Can you work these out from the model? Positions are in its coordinate system, mm. Face numbers are marked on the shaded views. A direction names the side the tool comes from. Give positions to 0.01 mm unless a question says otherwise; leave off trailing zeros. Write each loop counter-clockwise with the first axis right and the second up, starting at its lowest first coordinate (ties: lowest second). Pieces come first, ordered by that corner, then holes. Notation, with made-up numbers: M 86,-10.5 L 133,-10.5 A19 cw 133,26.5 Z; hole C 84,8.25 d2. An arc over 180 degrees is marked long. Use CSV: the item, a comma, the result in double quotes. Start each with the question number.
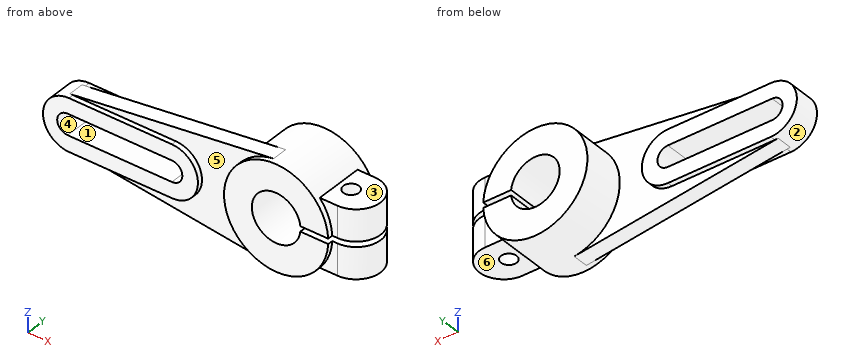
from build123d import *

# Parameters (mm, degrees)
BOSS_EXTRUDE1_DEPTH = 7.5
BOSS_EXTRUDE2_DEPTH = 4.5
BOSS_EXTRUDE3_START = 28.5
BOSS_EXTRUDE3_DEPTH = 36
BOSS_EXTRUDE4_START = 23.5
SKETCH1_5_W         = 16.939679335
SKETCH1_5_H         = 18
BOSS_EXTRUDE4_DEPTH = 28
FILLET1_RADIUS      = 14
FILLET1_LENGTH      = 18
FILLET2_RADIUS      = 14
FILLET2_LENGTH      = 18
SKETCH2_R           = 4.5
CUT_EXTRUDE1_DEPTH  = 146.8618303


with BuildPart() as part:
    # Sketch1 → Boss-Extrude1 (new, symmetric)
    with BuildSketch(Plane(origin=(0, 0, 0), x_dir=(1, 0, 0), z_dir=(0, 1, 0))):
        with BuildLine():
            Line((-119.21316455, -15), (-60, -15))
            ThreePointArc((-60, -15), (-45, 0), (-60, 15))
            Line((-60, 15), (-119.21316455, 15))
            ThreePointArc((-119.21316455, 15), (-134.21316455, 0), (-119.21316455, -15))
        make_face()
        with BuildLine():
            ThreePointArc((-120, 6), (-126, 0), (-120, -6))
            Line((-120, -6), (-60, -6))
            ThreePointArc((-60, -6), (-54, 0), (-60, 6))
            Line((-60, 6), (-120, 6))
        make_face(mode=Mode.SUBTRACT)
    extrude(amount=BOSS_EXTRUDE1_DEPTH, both=True)

    # Sketch1<3> → Boss-Extrude2 (add, symmetric)
    with BuildSketch(Plane(origin=(0, 0, 0), x_dir=(1, 0, 0), z_dir=(0, 1, 0))):
        with BuildLine():
            ThreePointArc((-121.100539999, 14.880786737), (-120.158732883, 14.970167017), (-119.21316455, 15))
            Line((-119.21316455, 15), (-60, 15))
            ThreePointArc((-60, 15), (-45, 0), (-60, -15))
            Line((-60, -15), (-119.21316455, -15))
            ThreePointArc((-119.21316455, -15), (-120.158732883, -14.970167017), (-121.100539999, -14.880786737))
            Line((-121.100539999, -14.880786737), (-3.774750899, -29.761573474))
            ThreePointArc((-3.774750899, -29.761573474), (-30, 0), (-3.774750899, 29.761573474))
            Line((-3.774750899, 29.761573474), (-121.100539999, 14.880786737))
        make_face()
    extrude(amount=BOSS_EXTRUDE2_DEPTH, both=True)

    # Sketch1<4> → Boss-Extrude3 (add)
    with BuildSketch(Plane(origin=(0, 0, 0), x_dir=(1, 0, 0), z_dir=(0, 1, 0)).offset(BOSS_EXTRUDE3_START)):
        with BuildLine():
            ThreePointArc((29.962476533, 1.5), (-30, 0), (29.962476533, -1.5))
            Line((29.962476533, -1.5), (13.919410907, -1.5))
            ThreePointArc((13.919410907, -1.5), (-14, 0), (13.919410907, 1.5))
            Line((13.919410907, 1.5), (29.962476533, 1.5))
        make_face()
    extrude(amount=-BOSS_EXTRUDE3_DEPTH)

    # Sketch1<5> → Boss-Extrude4 (add)
    with BuildSketch(Plane(origin=(0, 0, 0), x_dir=(1, 0, 0), z_dir=(0, 1, 0)).offset(BOSS_EXTRUDE4_START)):
        with BuildLine():
            ThreePointArc((29.962476533, -1.5), (27.873242778, -11.094247926), (22.79802623, -19.5))
            Line((22.79802623, -19.5), (29.962476533, -19.5))
            Line((29.962476533, -19.5), (29.962476533, -1.5))
        make_face()
        with Locations((38.4323162, -10.5)):
            Rectangle(SKETCH1_5_W, SKETCH1_5_H)
        with Locations((38.4323162, 10.5)):
            Rectangle(SKETCH1_5_W, SKETCH1_5_H)
        with BuildLine():
            Line((29.962476533, 19.5), (22.79802623, 19.5))
            ThreePointArc((22.79802623, 19.5), (27.873242778, 11.094247926), (29.962476533, 1.5))
            Line((29.962476533, 1.5), (29.962476533, 19.5))
        make_face()
    extrude(amount=-BOSS_EXTRUDE4_DEPTH)

    # Fillet1: full round fillet: the end face becomes a half cylinder, R = half its width
    fillet1_face = Plane((46.902155868, 9.5, 10.5), x_dir=(0, 0, -1), z_dir=(1, 0, 0))  # on the end face: x along it, z out of the body
    fillet1_slab = fillet1_face.offset(-FILLET1_RADIUS / 2) * Box(FILLET1_LENGTH, 2 * FILLET1_RADIUS, FILLET1_RADIUS, mode=Mode.PRIVATE)  # the body's end, R deep
    fillet1_round = Plane((32.902155868, 9.5, 10.5), x_dir=(1, 0, 0), z_dir=(0, 0, -1)) * Cylinder(FILLET1_RADIUS, FILLET1_LENGTH, mode=Mode.PRIVATE)  # its axis R under the face
    add(fillet1_slab - fillet1_round, mode=Mode.SUBTRACT)

    # Fillet2: full round fillet: the end face becomes a half cylinder, R = half its width
    fillet2_face = Plane((46.902155868, 9.5, -10.5), x_dir=(0, 0, 1), z_dir=(1, 0, 0))  # on the end face: x along it, z out of the body
    fillet2_slab = fillet2_face.offset(-FILLET2_RADIUS / 2) * Box(FILLET2_LENGTH, 2 * FILLET2_RADIUS, FILLET2_RADIUS, mode=Mode.PRIVATE)  # the body's end, R deep
    fillet2_round = Plane((32.902155868, 9.5, -10.5), x_dir=(1, 0, 0), z_dir=(0, 0, 1)) * Cylinder(FILLET2_RADIUS, FILLET2_LENGTH, mode=Mode.PRIVATE)  # its axis R under the face
    add(fillet2_slab - fillet2_round, mode=Mode.SUBTRACT)

    # Sketch2 → Cut-Extrude1 (cut, through all)
    with BuildSketch(Plane.XY.offset(19.5)):
        with Locations(Location((29.962476533, 9.5, 0), (0, 0, 180))):
            Circle(SKETCH2_R)
    extrude(amount=-CUT_EXTRUDE1_DEPTH, mode=Mode.SUBTRACT)


solid = part.part
(1) Which directions (+Z, -Z, +X, -X, +Y, -Y) give clear straight access to the entire face, cutting with the end or side of a thin tool? Please do the marked faces 4, 5 and 6.
(2) Please list where these lines run through material, in increasing order: L1, parallel to Z at x = 0, y = 9.5; L2, parallel to X at y = 6, z = 9.5; L3, parallel to Z at x = -60, y = 7. Write a range as [from, to].
(3) I want a section at A-A (y = 9.5). Write out the boundary of the cut face in (x, z).
(4) I want a section at B-B (x = 0). Write out the boundary of the cut face in (y, z), and give its area (3 significant figures).
(5) Thinking about a two-plate mould opening in Z: for the marked faces 1, 2 and 3, which applies, released by +Z, released by -Z, zero draft, split by the parting line, or undercut?
(6) I want a section at D-D (y = 2). Write out the boundary of the cut face in (x, z).
(7) I want a section at C-C (x = -111.5). Write out the boundary of the cut face in (y, z).
(8) Will these pins go through, and if not, where does the flat tip stop? pin 1 Ø2 at (x, y) = (22.5, 8) entering from -Z; pin 2 Ø8 at (y, z) = (-2, 17.5) entering from +X; pin 3 Ø19.5 at (x, y) = (31, 4.5) entering from -Z; pin 4 Ø7 at (x, y) = (29.96, 9.5) entering from -Z.
Geometry results:
1,face 4,"+Y, -Y"
1,face 5,"-Y"
1,face 6,"-Z, +X, +Y, -Y"
2,L1,"z = [-30, -14], [14, 30]"
2,L2,"x = [-130.82, -48.39], [-28.46, -10.28], [10.28, 27.13], [32.79, 46.46]"
2,L3,"z = [-15, -6], [6, 15]"
3,outline,"M 13.92,-1.5 A14 cw long 13.92,1.5 L 25.46,1.5 L 25.46,19.5 L 22.8,19.5 A30 ccw long 22.8,-19.5 L 25.46,-19.5 L 25.46,-1.5 Z; M 34.46,-19.5 L 46.9,-19.5 L 46.9,-1.5 L 34.46,-1.5 Z; M 34.46,1.5 L 46.9,1.5 L 46.9,19.5 L 34.46,19.5 Z"
4,outline,"M -7.5,-30 L 28.5,-30 L 28.5,-14 L -7.5,-14 Z; M -7.5,14 L 28.5,14 L 28.5,30 L -7.5,30 Z"
4,area,"1,150 mm2"
5,face 1,"undercut"
5,face 2,"split by the parting line"
5,face 3,"released by +Z"
6,outline,"M -121.1,-14.88 L -3.77,-29.76 A30 ccw 22.8,-19.5 L 44.72,-19.5 L 44.72,-1.5 L 13.92,-1.5 A14 cw long 13.92,1.5 L 44.72,1.5 L 44.72,19.5 L 22.8,19.5 A30 ccw -3.77,29.76 L -121.1,14.88 A15 ccw Z; hole M -120,-6 L -60,-6 A6 ccw -60,6 L -120,6 A6 ccw Z"
7,outline,"M -7.5,-15 L -4.5,-15 L -4.5,-16.1 L 4.5,-16.1 L 4.5,-15 L 7.5,-15 L 7.5,-6 L -7.5,-6 Z; M -7.5,6 L 7.5,6 L 7.5,15 L 4.5,15 L 4.5,16.1 L -4.5,16.1 L -4.5,15 L -7.5,15 Z"
8,pin 1,"stops at z = -20.92"
8,pin 2,"stops at x = 44.72"
8,pin 3,"stops at z = -21.18"
8,pin 4,"passes through"
